Could you check a few things on this model? Use its own coordinates, in mm. A direction names the side the tool comes from. Coordinates: 2 decimals unless noted, no trailing zeros. Write each loop counter-clockwise with the first axis right and the second up, starting at its lowest first coordinate (ties: lowest second). Pieces come first, ordered by that corner, then holes.
```python
from build123d import *

# Parameters (mm, degrees)
F0_W     = 360
F0_H     = 360
F1_DEPTH = 600
F2_R     = 4
F3_DEPTH = 406
F4_R     = 4
F5_DEPTH = 467


with BuildPart() as f1:
    # F0 (on Top) → F1 (new body)
    with BuildSketch(Plane.XY):
        Polygon((0, 400), (0, 0), (20, 0), (400, 0), (400, 400), align=None)
        with Locations((200, 200)):
            Rectangle(F0_W, F0_H, mode=Mode.SUBTRACT)
    extrude(amount=F1_DEPTH)

    # F2 (on face) → F3 (cut)
    with BuildSketch(Plane.XZ):
        with Locations((37.5, 560)):
            Circle(F2_R)
        with BuildLine():
            ThreePointArc((366.5, 560), (362.5, 564), (358.5, 560))
            ThreePointArc((358.5, 560), (362.5, 556), (366.5, 560))
        make_face()
    extrude(amount=-F3_DEPTH, mode=Mode.SUBTRACT)

    # F4 (on face) → F5 (cut)
    with BuildSketch(Plane(origin=(0, 0, 0), x_dir=(0, -1, 0), z_dir=(-1, 0, 0))):
        with Locations((-362.5, 535)):
            Circle(F4_R)
        with BuildLine():
            ThreePointArc((-33.5, 535), (-37.5, 539), (-41.5, 535))
            ThreePointArc((-41.5, 535), (-37.5, 531), (-33.5, 535))
        make_face()
    extrude(amount=-F5_DEPTH, mode=Mode.SUBTRACT)


solid = f1.part
```
1. Please list where these lines run through material, in increasing order: line 1 along Y through (x, z) = (15.5, 535); line 2 along X through (y, z) = (348, 73.5).
Verdict:
line 1: y = 0 to 33.5, 41.5 to 358.5, 366.5 to 400
line 2: x = 0 to 20, 380 to 400
2. If we mould it in two halves opening along Y, with no side actions, what happens to faces 3 (the face through (203, 400, 296)), 4 (the face through (400, 197, 296)), 5 (the face through (197, 20, 296)), 6 (the face through (197, 380, 296))? For each: pulls with the +Y half, pulls with the -Y half, needs draft (parallel to the pull), parting line crosses it, or undercut.
Verdict:
face 3: pulls with the +Y half
face 4: needs draft
face 5: undercut
face 6: undercut
3. I want a section at A-A on y = 74.5. Please give me the cut outline in (x, z).
Verdict:
outline: (0, 0) - (20, 0) - (20, 600) - (0, 600) - close; (380, 0) - (400, 0) - (400, 600) - (380, 600) - close
4. On a 3-axis mill with a long thin cutter (end or side, diameter ignored), from which of +Z, -Z, +X, -X, +Y, -Y can I reach the whole of each face in a straight line? I mean faces 1 (the face through (380, 197, 296)), 2 (the face through (0, 203, 296)). Say none if no direction works.
Verdict:
face 1: +Z, -Z
face 2: +Z, -Z, -X, +Y, -Y
5. For pin 1 (10.5 mm diameter, centred on y = 362.5, z = 535, fed in from -X); pin 2 (6.5 mm diameter, centred on x = 37.5, z = 560, fed in from +Y), each with a flat end and sliding along its axis, tell me the tip position at first contact or that it passes through.
Verdict:
pin 1: stops at x = 0
pin 2: passes through
6. I want a section at C-C on z = 49.5. Please give me the cut outline in (x, y), plus the area to 3 significant figures.
Verdict:
outline: (0, 0) - (400, 0) - (400, 400) - (0, 400) - close; hole (20, 20) - (380, 20) - (380, 380) - (20, 380) - close
area: 30,400 mm2
